CAD build for the part. Positions are in the model's coordinates, mm. A direction names the side the tool comes from. Coordinates: 2 decimals unless noted, no trailing zeros. Loops run counter-clockwise (first coordinate to the right, second up) from the corner with the lowest first, then second, coordinate; pieces in that order, holes last. Notation, with made-up numbers: (-24.5, 54.25) -> (4.5, 54.25) arc R36 cw to (4.5, 93.25) -> close; hole circle Ø3 at (54, 70.25). An arc over 180 degrees is marked (long way). Write item = value, one per line. Start each with the question number.
(1) Band-saw the part on B-B (x = 0). Write the cut outline in (y, z), and give its area (3 significant figures).
(2) Drill centre lines: line 1 (Y direction, x = 0, z = -2); line 2 (Y direction, x = 4.5, z = -3.25); line 3 (X direction, y = 23, z = -7.25). Where is each one in solid material? Low to high. Write a range as from..to.
(3) Band-saw the part on C-C (z = -6.5). Write the cut outline in (x, y).
(4) Band-saw the part on A-A (y = -31.75). Write the cut outline in (x, z), and give its area (3 significant figures).
(5) Tool access for faces 4 (the face through (-108, 25.4, 0)), 5 (the face through (-101.6, 67, 0)), 6 (the face through (101.6, -13, 0)), 7 (the face through (24, 1, -12.7)), 8 (the face through (101.6, 67, 0)): list every direction of +Z, -Z, +X, -X, +Y, -Y with a clear straight run to the whole face (end or side of a thin tool).
(6) Pull direction Y, two halves, no side cores. Call faces 1 (the face through (90.14, -78.04, 0.18)), 2 (the face through (-1.653, 76.092, -0.171)), 3 (the face through (-108, 50.8, 0)): +Y half, -Y half, draft (parallel to the pull), parting line (faces both ways), or undercut.
(7) Band-saw the part on D-D (y = 63.5). Write the cut outline in (x, z), and give its area (3 significant figures).
(8) Flat gauge pins, fed straight in: P1, Ø4, axis at x = 107.5, z = 5, coming from the -Y side; P2, Ø10, axis at x = 106, z = -1, coming from the +Y side (3 decimals); P3, Ø7.5, axis at y = 64.5, z = -2.5, coming from the -X side. Where does each tip first touch, or does it go through?
```python
from build123d import *

# Parameters (mm, degrees)
F0_W     = 203.2
F0_H     = 177.8
F0_R     = 38.1
F0_R_2   = 12.7
F1_DEPTH = 12.7
F2_SIZE  = 0.508
F3_SIZE  = 1.524
F4_R     = 38.1
F5_R     = 5.08
F6_W     = 12.7
F6_H     = 25.4
F7_DEPTH = 25.4


with BuildPart() as f1:
    # F0 (on Top) → F1 (new body, symmetric)
    with BuildSketch(Plane.XY):
        Rectangle(F0_W, F0_H)
        with Locations((0, -31.75)):
            Circle(F0_R, mode=Mode.SUBTRACT)
        with Locations((0, 63.5)):
            Circle(F0_R_2, mode=Mode.SUBTRACT)
    extrude(amount=F1_DEPTH, both=True)

    # F2
    f2_edges = [f1.edges().sort_by_distance(p)[0] for p in [
        (-12.7, 63.5, 12.7),
        (-12.7, 63.5, -12.7),
    ]]
    chamfer(f2_edges, length=F2_SIZE)

    # F3
    f3_edges = [f1.edges().sort_by_distance(p)[0] for p in [
        (-38.1, -31.75, 12.7),
        (-38.1, -31.75, -12.7),
    ]]
    chamfer(f3_edges, length=F3_SIZE)

    # F4
    f4_edges = [f1.edges().sort_by_distance(p)[0] for p in [
        (-101.6, -88.9, 0),
        (101.6, -88.9, 0),
    ]]
    fillet(f4_edges, radius=F4_R)

    # F5
    f5_edges = [f1.edges().sort_by_distance(p)[0] for p in [
        (101.6, 88.9, 0),
        (-101.6, 88.9, 0),
    ]]
    fillet(f5_edges, radius=F5_R)

    # F6 (on face) → F7 (join)
    with BuildSketch(Plane.XY.offset(12.7)):
        with Locations((-107.95, 38.1)):
            Rectangle(F6_W, F6_H)
        with Locations((107.95, 38.1)):
            Rectangle(F6_W, F6_H)
    extrude(amount=-F7_DEPTH)


solid = f1.part
```
Findings below:
q1.outline = (-88.9, -12.7) -> (-71.37, -12.7) -> (-69.85, -11.18) -> (-69.85, 11.18) -> (-71.37, 12.7) -> (-88.9, 12.7) -> close; (6.35, -11.18) -> (7.87, -12.7) -> (50.29, -12.7) -> (50.8, -12.19) -> (50.8, 12.19) -> (50.29, 12.7) -> (7.87, 12.7) -> (6.35, 11.18) -> close; (76.2, -12.19) -> (76.71, -12.7) -> (88.9, -12.7) -> (88.9, 12.7) -> (76.71, 12.7) -> (76.2, 12.19) -> close
q1.area = 1,930 mm²
q2.line_1 = -88.9..-69.85, 6.35..50.8, 76.2..88.9
q2.line_2 = -88.9..-69.58, 6.08..51.62, 75.38..88.9
q2.line_3 = -101.6..101.6
q3.outline = (-114.3, 25.4) -> (-101.6, 25.4) -> (-101.6, -50.8) arc R38.1 ccw to (-63.5, -88.9) -> (63.5, -88.9) arc R38.1 ccw to (101.6, -50.8) -> (101.6, 25.4) -> (114.3, 25.4) -> (114.3, 50.8) -> (101.6, 50.8) -> (101.6, 83.82) arc R5.08 ccw to (96.52, 88.9) -> (-96.52, 88.9) arc R5.08 ccw to (-101.6, 83.82) -> (-101.6, 50.8) -> (-114.3, 50.8) -> close; hole circle Ø76.2 at (0, -31.75); hole circle Ø25.4 at (0, 63.5)
q4.outline = (-101.6, -12.7) -> (-39.62, -12.7) -> (-38.1, -11.18) -> (-38.1, 11.18) -> (-39.62, 12.7) -> (-101.6, 12.7) -> close; (38.1, -11.18) -> (39.62, -12.7) -> (101.6, -12.7) -> (101.6, 12.7) -> (39.62, 12.7) -> (38.1, 11.18) -> close
q4.area = 3,220 mm²
q5.face_4 = +Z, -Z, -X, -Y
q5.face_5 = +Z, -Z, -X, +Y
q5.face_6 = +Z, -Z, +X, -Y
q5.face_7 = -Z, +X, -X, +Y, -Y
q5.face_8 = +Z, -Z, +X, +Y
q6.face_1 = -Y half
q6.face_2 = undercut
q6.face_3 = +Y half
q7.outline = (-101.6, -12.7) -> (-13.21, -12.7) -> (-12.7, -12.19) -> (-12.7, 12.19) -> (-13.21, 12.7) -> (-101.6, 12.7) -> close; (12.7, -12.19) -> (13.21, -12.7) -> (101.6, -12.7) -> (101.6, 12.7) -> (13.21, 12.7) -> (12.7, 12.19) -> close
q7.area = 4,520 mm²
q8.P1 = 25.4
q8.P2 = 86.215
q8.P3 = -101.6
